from build123d import *

# Parameters (mm, degrees)
F1_DEPTH  = 40
F5_D      = 2.2606
F5_DEPTH  = 3.071
F6_D      = 2.2606
F7_D      = 2.2606
F7_DEPTH  = 3.071
F8_D      = 2.2606
F11_D     = 5.1054
F11_DEPTH = 3.048
F11_TIP   = 1.5338169022
F12_D     = 5.1054
F12_DEPTH = 3.048
F12_TIP   = 1.5338169022


with BuildPart() as f1:
    # F0 (on Front) → F1 (new body, symmetric)
    with BuildSketch(Plane.XZ):
        Polygon((-7.8, 3.07), (-10.6, 0.27), (-10.6, -0.27), (-7.8, -3.07), (7.8, -3.07), (10.6, -0.27), (10.6, 0.27), (7.8, 3.07), align=None)
    extrude(amount=F1_DEPTH, both=True)

    # F5 (through all, one way)
    with BuildSketch(Plane.XY):
        with Locations((0, -35)):
            Circle(F5_D / 2)
    extrude(amount=-F5_DEPTH, mode=Mode.SUBTRACT)

    # F6 (through all)
    with Locations(Plane(origin=(0, 0, 0), x_dir=(1, 0, 0), z_dir=(0, 0, -1))):
        with Locations((0, 35)):
            Hole(F6_D / 2)

    # F7 (through all, one way)
    with BuildSketch(Plane.XY):
        with Locations((0, 35)):
            Circle(F7_D / 2)
    extrude(amount=-F7_DEPTH, mode=Mode.SUBTRACT)

    # F8 (through all)
    with Locations(Plane(origin=(0, 0, 0), x_dir=(1, 0, 0), z_dir=(0, 0, -1))):
        with Locations((0, -35)):
            Hole(F8_D / 2)

    # F11
    with Locations(Plane(origin=(0, 0, -3.07), x_dir=(1, 0, 0), z_dir=(0, 0, -1))):
        with Locations((0, 35)):
            Hole(F11_D / 2, depth=F11_DEPTH)
            with Locations((0, 0, -(F11_DEPTH + F11_TIP / 2))):  # 118° drill point
                Cone(0, F11_D / 2, F11_TIP, mode=Mode.SUBTRACT)

    # F12 (one way)
    with BuildSketch(Plane.XY):
        with Locations((0, 35)):
            Circle(F12_D / 2)
    extrude(amount=-F12_DEPTH, mode=Mode.SUBTRACT)
    with Locations(Plane.XY):
        with Locations((0, 35)):
            with Locations((0, 0, -(F12_DEPTH + F12_TIP / 2))):  # 118° drill point
                Cone(0, F12_D / 2, F12_TIP, mode=Mode.SUBTRACT)


solid = f1.part
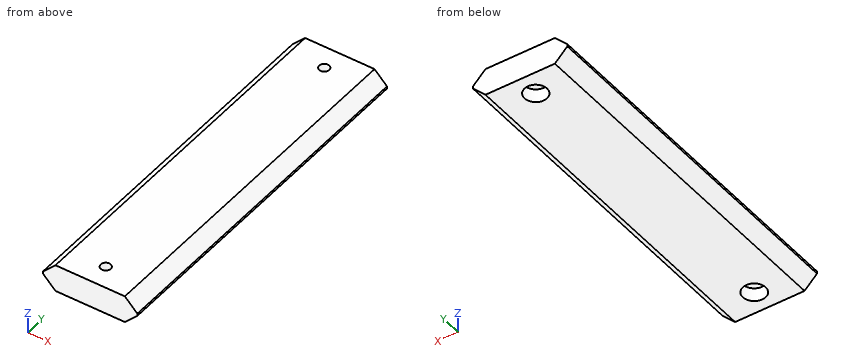
Here's how the part is built. I have some questions about the finished solid (model axes, mm). Give positions to 0.01 mm unless a question says otherwise; leave off trailing zeros. Order: outer loops, then holes, each group sorted by start corner. A loop starts at its lowest first (then second) coordinate and runs counter-clockwise, first axis right, second up. Notation, with made-up numbers: (66, 31) -> (106, 31) arc R16 ccw to (106, 60) -> close; hole circle Ø10 at (9.5, 63.5). An arc over 180 degrees is marked (long way). Use a Markdown table: item, result. Add a question column.
Item 1: Will these pins go through, and if not, where does the flat tip stop? pin 1 (1 mm diameter, centred on y = -28.5, z = 1, fed in from -X); pin 2 (4.5 mm diameter, centred on x = 0, y = -35, fed in from -Z); pin 3 (4.5 mm diameter, centred on x = 0, y = 35, fed in from -Z).
Item 2: Imagine slicing it at D-D on x = 0. Please give me the cut outline in (y, z), plus the area to 3 significant figures.
Item 3: Imagine slicing it at A-A on y = -35. Please give me the cut outline in (x, z).
Item 4: I need wall thicknesses on line 1 (Y direction, x = 0, z = -1.6); line 2 (Y direction, x = 0, z = 2.35); line 3 (X direction, y = 35, z = 1.15). Which ranges of each line are inside material? Lowest first, please.
Item 5: Imagine slicing it at B-B on z = 1.75. Please give me the cut outline in (x, y).
Item 6: Imagine slicing it at C-C on y = 4. Please give me the cut outline in (x, z).
Data:
| question | item | result |
|---|---|---|
| 1 | pin 1 | stops at x = -10.37 |
| 1 | pin 2 | stops at z = 0.16 |
| 1 | pin 3 | stops at z = 0 |
| 2 | outline | (-40, -3.07) -> (-37.55, -3.07) -> (-37.55, -0.02) -> (-36.13, 0.83) -> (-36.13, 3.07) -> (-40, 3.07) -> close; (-33.87, 0.83) -> (-32.45, -0.02) -> (-32.45, -3.07) -> (32.48, -3.07) -> (32.45, -3.05) -> (32.45, 0) -> (33.87, 0) -> (33.87, 3.07) -> (-33.87, 3.07) -> close; (36.13, 0) -> (37.55, 0) -> (37.55, -3.05) -> (37.52, -3.07) -> (40, -3.07) -> (40, 3.07) -> (36.13, 3.07) -> close |
| 2 | area | 445 mm² |
| 3 | outline | (-10.6, -0.27) -> (-7.8, -3.07) -> (-2.55, -3.07) -> (-2.55, -0.02) -> (-1.13, 0.83) -> (-1.13, 3.07) -> (-7.8, 3.07) -> (-10.6, 0.27) -> close; (1.13, 0.83) -> (2.55, -0.02) -> (2.55, -3.07) -> (7.8, -3.07) -> (10.6, -0.27) -> (10.6, 0.27) -> (7.8, 3.07) -> (1.13, 3.07) -> close |
| 4 | line 1 | y = -40 to -37.55, -32.45 to 32.45, 37.55 to 40 |
| 4 | line 2 | y = -40 to -36.13, -33.87 to 33.87, 36.13 to 40 |
| 4 | line 3 | x = -9.72 to -1.13, 1.13 to 9.72 |
| 5 | outline | (-9.12, -40) -> (9.12, -40) -> (9.12, 40) -> (-9.12, 40) -> close; hole circle Ø2.26 at (0, -35); hole circle Ø2.26 at (0, 35) |
| 6 | outline | (-10.6, -0.27) -> (-7.8, -3.07) -> (7.8, -3.07) -> (10.6, -0.27) -> (10.6, 0.27) -> (7.8, 3.07) -> (-7.8, 3.07) -> (-10.6, 0.27) -> close |
